Check sheet for the drawn part. Datum: minimum x, y, z corner. Units: mm. A direction names the side the tool comes from. Round coordinates to 2 decimals unless told otherwise and drop trailing zeros. Write each loop counter-clockwise with the first axis right and the second up, starting at its lowest first coordinate (ties: lowest second). Pieces come first, ordered by that corner, then holes.
Item 1: Release check for a two-part mould opening along Z. For the marked faces 4, 5, 6 and 7 record: +Z half, -Z half, draft (parallel to the pull), parting line (faces both ways), or undercut.
Item 2: Tool access check on the marked faces 1, 2 and 3. Record the directions out of +Z, -Z, +X, -X, +Y, -Y that give a thin tool (end or side, any length) a straight path to the whole face; none if there is none.
Item 3: Cross-section at C-C on x = 10.25. Enter the section's corners in (y, z), plus the area to 3 significant figures.
Item 4: Cross-section at B-B on y = 32.5. Enter the section's corners in (x, z), plus the area to 3 significant figures.
Item 5: Material ranges on line 1 (Y direction, x = 9.25, z = 14); line 2 (Z direction, x = 5.75, y = 35); line 3 (Z direction, x = 8, y = 8.5), recorded low to high.
Item 6: Cross-section at D-D on z = 4.5. Enter the section's corners in (x, y).
Item 7: Go/stop test with flat-tipped pins: pin 1 Ø12 at (y, z) = (24.5, 12.5) entering from -X; pin 2 Ø1.5 at (x, z) = (5.5, 31.5) entering from +Y; pin 3 Ø3.5 at (x, y) = (6, 19) entering from +Z; pin 4 Ø6 at (x, y) = (2.5, 31) entering from -Z. Record where each tip stops, or that it passes through.
Item 8: Cross-section at A-A on z = 15.5. Enter the section's corners in (x, y).
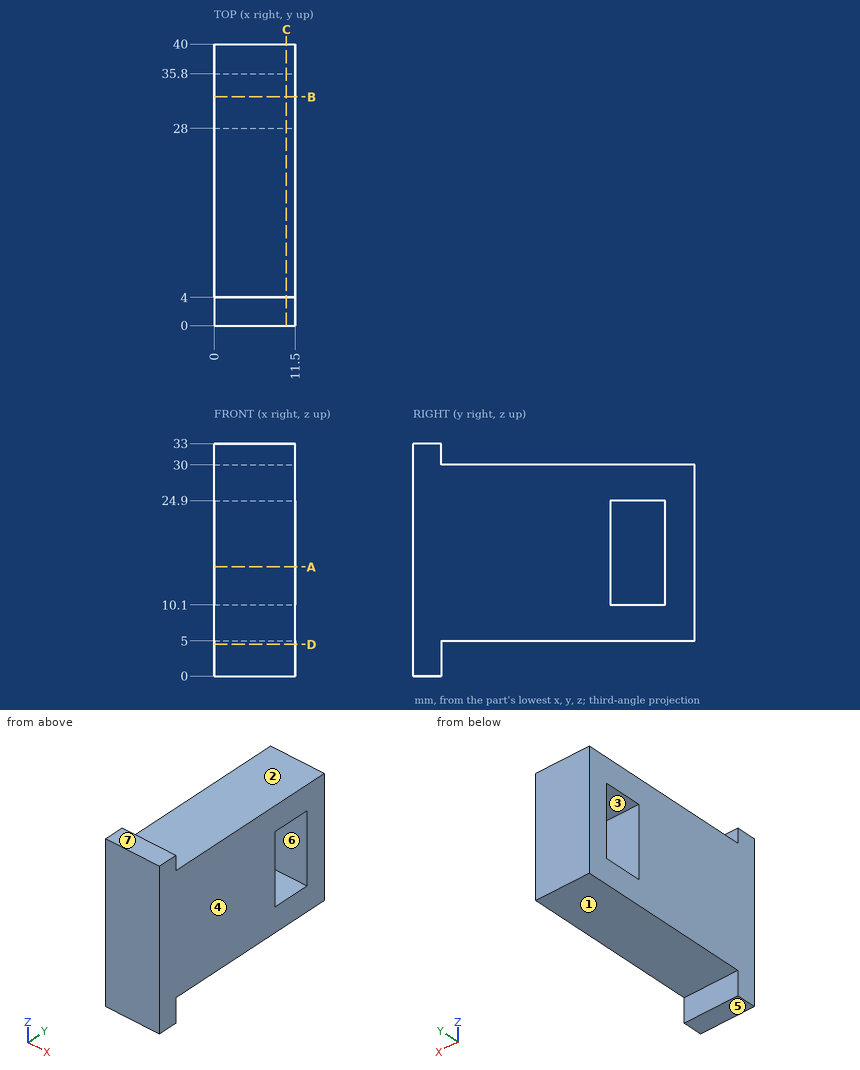
Response values:
1. face 4: draft
1. face 5: -Z half
1. face 6: undercut
1. face 7: +Z half
2. face 1: -Z, +X, -X, +Y
2. face 2: +Z, +X, -X, +Y
2. face 3: +X, -X
3. outline: (0, 0) - (4, 0) - (4, 5) - (40, 5) - (40, 30) - (4, 30) - (4, 33) - (0, 33) - close; hole (28, 10.1) - (35.8, 10.1) - (35.8, 24.9) - (28, 24.9) - close
3. area: 917 mm2
4. outline: (0, 5) - (11.5, 5) - (11.5, 10.1) - (0, 10.1) - close; (0, 24.9) - (11.5, 24.9) - (11.5, 30) - (0, 30) - close
4. area: 117 mm2
5. line 1: y = 0 to 28, 35.8 to 40
5. line 2: z = 5 to 10.1, 24.9 to 30
5. line 3: z = 5 to 30
6. outline: (0, 0) - (11.5, 0) - (11.5, 4) - (0, 4) - close
7. pin 1: stops at x = 0
7. pin 2: stops at y = 4
7. pin 3: stops at z = 30
7. pin 4: stops at z = 5
8. outline: (0, 0) - (11.5, 0) - (11.5, 28) - (0, 28) - close; (0, 35.8) - (11.5, 35.8) - (11.5, 40) - (0, 40) - close
